Work out the finished part from the listing and answer in its coordinate system (mm). Face numbers are marked on the shaded views. A direction names the side the tool comes from. Coordinates: 2 decimals unless noted, no trailing zeros. Write each loop counter-clockwise with the first axis right and the second up, starting at its lowest first coordinate (ties: lowest second). Pieces come first, ordered by that corner, then holes. Notation, with made-up numbers: (62.25, 72.5) - (109.25, 72.5) arc R29 ccw to (109.25, 107.5) - close; hole circle Ø9 at (67, 43.25). An arc over 180 degrees is marked (long way). One line per item, written item: value.
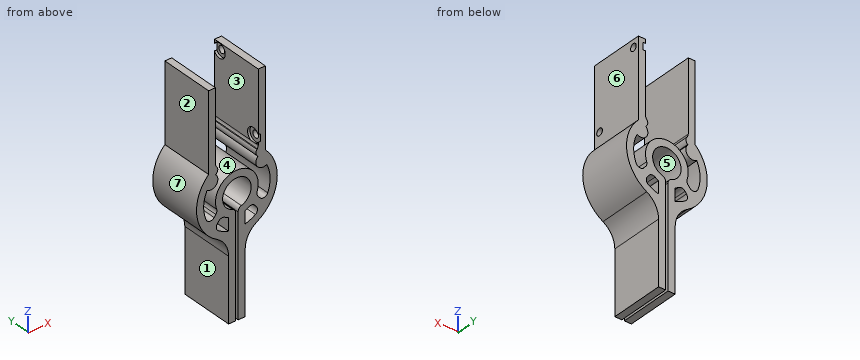
Autodesk Inventor part; units mm, degrees
ref_plane "YZ Plane" through (0, 0, 0) normal (1, 0, 0) x (0, 1, 0)
ref_plane "XZ Plane" through (0, 0, 0) normal (0, 1, 0) x (-1, 0, 0)
ref_plane "XY Plane" through (0, 0, 0) normal (0, 0, 1) x (1, 0, 0)
sketch "Sketch1" plane through (0, 0, 0) normal (0, 1, 0) x (-1, 0, 0)
  line L0 (3, 0) -> (3, -26.9193)
  line L1 (0, -30) -> (0, 0)
  line L2 (3, 0) -> (3, 3)
  line L3 (3, 3) -> (0, 3)
  line L4 (0, 3) -> (0, 0)
  line L5 (21, 0) -> (21, -26.9193)
  line L6 (23.8993, -30) -> (23.8993, -0.0434)
  line L7 (21, 0) -> (21, 3)
  line L8 (21, 3) -> (23.8993, 3)
  line L9 (23.8993, 3) -> (23.8993, -0.0434)
  line L10 (20.6088, -28.1075) -> (20.4284, -28.3517)
  line L11 (3.3912, -28.1075) -> (3.5716, -28.3517)
  arc A0 (13.875, -47.6995) -> (10.125, -47.6995) centre (12, -42) ccw
  line L12 (12.5, -49.5993) -> (12.5, -92)
  line L13 (12.5, -92) -> (15.5, -92)
  line L14 (11.5, -49.5993) -> (11.5, -92)
  line L15 (11.5, -92) -> (8.5, -92)
  arc A1 (0, -29.9584) -> (3.5, -56.7224) centre (12, -42) ccw
  arc A2 (20.5, -56.7224) -> (23.8993, -29.8589) centre (12, -42) ccw
  line L16 (15.5, -92) -> (15.5, -65.3827)
  line L17 (15.5, -55.5554) -> (15.5, -50.2916)
  line L18 (8.5, -92) -> (8.5, -65.3827)
  line L19 (8.5, -55.5554) -> (8.5, -50.2916)
  arc A3 (20.9024, -31.195) -> (20.7826, -31.0974) centre (12, -42) ccw
  line L20 (19.6249, -49.9324) -> (20.2507, -50.7171)
  line L21 (23.8993, -51.3801) -> (24.2551, -51.0964)
  line L22 (21.5685, -47.7276) -> (20.8413, -46.8158)
  arc A4 (15.5, -55.5554) -> (19.8016, -53.6248) centre (12, -42) ccw
  arc A5 (24.9875, -47.2274) -> (24.5925, -35.8822) centre (12, -42) ccw
  arc A6 (15.5, -50.2916) -> (16.9592, -49.5104) centre (12, -42) ccw
  line L23 (4.3751, -49.9324) -> (3.7493, -50.7171)
  line L24 (2.4315, -47.7276) -> (3.1587, -46.8158)
  arc A7 (20.5132, -44.9199) -> (3.4868, -44.9199) centre (12, -42) ccw
  arc A8 (7.0408, -49.5104) -> (8.5, -50.2916) centre (12, -42) ccw
  arc A9 (4.1984, -53.6248) -> (8.5, -55.5554) centre (12, -42) ccw
  arc A10 (3.2174, -31.0974) -> (3.0976, -31.195) centre (12, -42) ccw
  arc A11 (-0.5925, -35.8822) -> (-0.9875, -47.2274) centre (12, -42) ccw
  arc A12 (20.5, -56.7224) -> (15.5, -65.3827) centre (25.5, -65.3827) ccw
  arc A13 (8.5, -65.3827) -> (3.5, -56.7224) centre (-1.5, -65.3827) ccw
  arc A14 (7.0408, -49.5104) -> (4.3751, -49.9324) centre (5.9387, -51.1794) ccw
  arc A15 (3.1587, -46.8158) -> (3.4868, -44.9199) centre (1.595, -45.5688) ccw
  arc A16 (-0.9875, -47.2274) -> (2.4315, -47.7276) centre (0.8679, -46.4806) ccw
  arc A17 (3.7493, -50.7171) -> (4.1984, -53.6248) centre (5.3129, -51.9641) ccw
  arc A18 (19.6249, -49.9324) -> (16.9592, -49.5104) centre (18.0613, -51.1794) ccw
  arc A19 (21.5685, -47.7276) -> (24.9875, -47.2274) centre (23.1321, -46.4806) ccw
  arc A20 (19.8016, -53.6248) -> (20.2507, -50.7171) centre (18.6871, -51.9641) ccw
  arc A21 (20.5132, -44.9199) -> (20.8413, -46.8158) centre (22.405, -45.5688) ccw
  arc A22 (3.2174, -31.0974) -> (3.5716, -28.3517) centre (1.9628, -29.5399) ccw
  arc A23 (20.4284, -28.3517) -> (20.7826, -31.0974) centre (22.0372, -29.5399) ccw
  arc A24 (20.6088, -28.1075) -> (21, -26.9193) centre (19, -26.9193) ccw
  arc A25 (3, -26.9193) -> (3.3912, -28.1075) centre (5, -26.9193) ccw
  arc A26 (13.875, -47.6995) -> (12.5, -49.5993) centre (14.5, -49.5993) ccw
  arc A27 (11.5, -49.5993) -> (10.125, -47.6995) centre (9.5, -49.5993) ccw
  arc A28 (20.9024, -31.195) -> (24.5925, -35.8822) centre (23, -33.3397) ccw
  arc A29 (-0.5925, -35.8822) -> (3.0976, -31.195) centre (1, -33.3397) ccw
  point P0 (19.2111, -30)
  point P1 (4.7889, -30)
  point P2 (12.5, -47.9791)
  point P3 (11.5, -47.9791)
  point P4 (8.5, -58.6358)
  point P5 (15.5, -58.6358)
  point P6 (18.3696, -48.3583)
  point P7 (21.4999, -52.2835)
  point P8 (23.4384, -50.0724)
  point P9 (20.1111, -45.9001)
  point P10 (5.6304, -48.3583)
  point P11 (2.5001, -52.2835)
  point P12 (0.5616, -50.0724)
  point P13 (3.8889, -45.9001)
  dimension "d4" = 3
  dimension "d6" = 3
  dimension "d7" = 3
  dimension "d8" = 90
  dimension "d9" = 10
  dimension "d10" = 2
  dimension "d11" = 2
  dimension "d12" = 2
  dimension "d13" = 6
  dimension "d14" = 6
extrude "Extrusion1" add sketch "Sketch1" along normal blind 23
sketch "Sketch3" plane through (-3, 0, -26.9193) normal (-1, 0, 0) x (0, 0, 1)
  line L0 (0, 23) -> (29.9193, 23)
  line L1 (29.9193, 23) -> (15.7246, 23)
  circle A0 centre (26.7681, 20.3773) radius 1.5
  circle A1 centre (26.7681, 20.3773) radius 3
  circle A2 centre (2.6381, 2.5973) radius 1.5
  circle A3 centre (2.6381, 2.5973) radius 3
  point P0 (26.9193, 0)
  point P1 (1.7246, 22.9923)
  point P2 (26.9193, 46)
  point P3 (1.7246, 23.0077)
extrude "Extrusion2" cut sketch "Sketch3" against normal blind 1 contours A1 L0 | L0 A1 | A0 | A2 | A3
extrude "Extrusion3" cut sketch "Sketch3" against normal blind 3 contours A0 | A2
Item 1: Which of the six approach directions +Z, -Z, +X, -X, +Y, -Y give full straight-line access (tool end or side, diameter ignored) to the marked faces 1, 2 and 3?
Evaluation:
face 1: -Z, -X, +Y, -Y
face 2: +Z, -X, +Y, -Y
face 3: +Z, +Y, -Y
Item 2: Determine the mould class of the marked faces 4, 5, 6 and 7 for opening direction Z: +Z half, -Z half, draft (parallel to the pull), parting line (faces both ways), or undercut.
Evaluation:
face 4: undercut
face 5: undercut
face 6: draft
face 7: parting line
Item 3: Section B-B, the plane z = -42 is taken. Determine the outline of the cut face in (x, y).
Evaluation:
outline: (-29, 0) - (-26, 0) - (-26, 23) - (-29, 23) - close; (-21, 0) - (-18, 0) - (-18, 23) - (-21, 23) - close; (-6, 0) - (-3, 0) - (-3, 23) - (-6, 23) - close; (2, 0) - (5, 0) - (5, 23) - (2, 23) - close
Item 4: Consider probe 1 along X at (y, z) = (13.25, -21); probe 2 along X at (y, z) = (1.5, -22); probe 3 along X at (y, z) = (5.5, -44.5). Determine where each line is inside the solid, lowest interval first.
Evaluation:
probe 1: x = -23.9 to -21, -3 to 0
probe 2: x = -23.9 to -21, -2 to 0
probe 3: x = -28.82 to -25.78, -20.65 to -17.45, -6.55 to -3.35, 1.77 to 4.82
Item 5: Section C-C, the plane z = -15.5 is taken. Determine the outline of the cut face in (x, y).
Evaluation:
outline: (-23.9, 0) - (-21, 0) - (-21, 23) - (-23.9, 23) - close; (-3, 0) - (0, 0) - (0, 23) - (-3, 23) - close
Item 6: Section A-A, the plane z = -76.5 is taken. Determine the outline of the cut face in (x, y), then the cut area to 3 significant figures.
Evaluation:
outline: (-15.5, 0) - (-12.5, 0) - (-12.5, 23) - (-15.5, 23) - close; (-11.5, 0) - (-8.5, 0) - (-8.5, 23) - (-11.5, 23) - close
area: 138 mm2
Item 7: Section D-D, the plane y = 14 is taken. Give the number of separate pieces and of enclosed holes in the cut face, then the cut area to 3 significant figures.
Evaluation:
separate pieces: 1
enclosed holes: 2
area: 869 mm2
Item 8: Given pin 1 (0.6 mm diameter, centred on y = 0.5, z = -26.5, fed in from -X); pin 2 (4 mm diameter, centred on x = -10, y = 10, fed in from +Z); pin 3 (9.5 mm diameter, centred on y = 20.38, z = -0.15, fed in from +X), each flat-ended and moving along its own axis, determine where each tip first touches the part or whether it passes through.
Evaluation:
pin 1: stops at x = -23.9
pin 2: stops at z = -33
pin 3: stops at x = 0
